Verification items for the finished model (mm, model axes). A direction names the side the tool comes from. Give positions to 0.01 mm unless a question says otherwise; leave off trailing zeros. Loops run counter-clockwise (first coordinate to the right, second up) from the corner with the lowest first, then second, coordinate; pieces in that order, holes last. Notation, with made-up numbers: (23, 3) - (50, 3) arc R21 ccw to (50, 35) - close; hole circle Ø8 at (-2, 53.25). An arc over 180 degrees is marked (long way). Use one line per item in the form item = value.
Autodesk Inventor part; units mm, degrees
ref_plane "YZ Plane" through (0, 0, 0) normal (1, 0, 0) x (0, 1, 0)
ref_plane "XZ Plane" through (0, 0, 0) normal (0, 1, 0) x (-1, 0, 0)
ref_plane "XY Plane" through (0, 0, 0) normal (0, 0, 1) x (1, 0, 0)
sketch "スケッチ1" plane through (0, 0, 0) normal (0, 0, 1) x (1, 0, 0)
  line L0 (-12.5, -43.5) -> (12.5, -43.5)
  line L1 (12.5, -43.5) -> (12.5, 43.5)
  line L2 (12.5, 43.5) -> (-12.5, 43.5)
  line L3 (-12.5, 43.5) -> (-12.5, -43.5)
  line L4 (-12.5, -43.5) -> (12.5, 43.5) construction
  line L5 (12.5, -43.5) -> (-12.5, 43.5) construction
  line L6 (9.6, -40.6) -> (-9.6, -40.6) construction
  line L7 (-9.6, -40.6) -> (-9.6, 40.6) construction
  line L8 (-9.6, 40.6) -> (9.6, 40.6) construction
  line L9 (9.6, 40.6) -> (9.6, -40.6) construction
  line L10 (9.6, -40.6) -> (-9.6, 40.6) construction
  line L11 (-9.6, -40.6) -> (9.6, 40.6) construction
  circle A0 centre (-9.6, -40.6) radius 1.6
  circle A1 centre (-9.6, 40.6) radius 1.6
  circle A2 centre (9.6, 40.6) radius 1.6
  circle A3 centre (9.6, -40.6) radius 1.6
  arc A4 (-7.4091, -42.5) -> (-11.5, -38.4091) centre (-9.6, -40.6) ccw
  line L12 (-7.4091, -42.5) -> (7.4091, -42.5)
  line L13 (0, -43.5) -> (0, 43.5) construction
  line L14 (-12.5, 0) -> (12.5, 0) construction
  arc A5 (11.5, -38.4091) -> (7.4091, -42.5) centre (9.6, -40.6) ccw
  arc A6 (-11.5, 38.4091) -> (-7.4091, 42.5) centre (-9.6, 40.6) ccw
  line L15 (-7.4091, 42.5) -> (7.4091, 42.5)
  arc A7 (7.4091, 42.5) -> (11.5, 38.4091) centre (9.6, 40.6) ccw
  line L16 (-11.5, -38.4091) -> (-11.5, 38.4091)
  line L17 (11.5, -38.4091) -> (11.5, 38.4091)
  point P0 (0, 0)
  dimension "d0" = 25
  dimension "d1" = 87
  dimension "d2" = 19.2
  dimension "d3" = 81.2
  dimension "d4" = 3.2
  dimension "d5" = 1
  dimension "d6" = 1
extrude "押し出し1" add sketch "スケッチ1" along normal blind 1.6 contours L3 L2 L1 L0 | A4 L16 A6 L15 A7 L17 A5 L12
extrude "押し出し2" add sketch "スケッチ1" along normal blind 9.34 contours A4 L16 A6 L15 A7 L17 A5 L12
fillet "フィレット1" radius 2 8 edges at (11.5, -38.4091, 5.47) (7.4091, -42.5, 5.47) (-7.4091, -42.5, 5.47) (-11.5, -38.4091, 5.47) (11.5, 38.4091, 5.47) (7.4091, 42.5, 5.47) (-7.4091, 42.5, 5.47) (-11.5, 38.4091, 5.47)
equation "\"d6\" = d5"
properties part number "IMU-Measurement-and-Transmission-Module"
1. Scan lines: probe 1 along Y at (x, z) = (9.6, 0.8); probe 2 along X at (y, z) = (-1.5, 5); probe 3 along Y at (x, z) = (4, 6). Record each from-to range of solid material in increasing order.
Result set:
probe_1 = -43.5 to -42.2, -39 to 39, 42.2 to 43.5
probe_2 = -11.5 to 11.5
probe_3 = -42.5 to 42.5
2. Tool access check on faces 1 (the cylindrical face through (6.12, 41.91, 5.52)), 2 (the flat face through (0, 42.5, 5)), 3 (the cylindrical face through (-6.12, -41.91, 5.52)). Record the directions out of +Z, -Z, +X, -X, +Y, -Y that give a thin tool (end or side, any length) a straight path to the whole face; none if there is none.
Result set:
face_1 = +Z, +X, +Y
face_2 = +Z, +X, -X, +Y
face_3 = +Z, -X, -Y
3. Draft check along Y on faces 4 (the flat face through (0, 1, 0)), 5 (the flat face through (0, -43.5, 1)), 6 (the cylindrical face through (-9.808, -42.186, 0.789)). Enter one of: released by +Y, released by -Y, zero draft, split by the parting line, or undercut.
Result set:
face_4 = zero draft
face_5 = released by -Y
face_6 = undercut
4. Section check B-B, the plane x = 0.25. Record the cut outline in (y, z).
Result set:
outline = (-43.5, 0) - (43.5, 0) - (43.5, 1.6) - (42.5, 1.6) - (42.5, 9.34) - (-42.5, 9.34) - (-42.5, 1.6) - (-43.5, 1.6) - close
5. Depth check by flat-ended pin: pin 1 Ø4 at (x, y) = (9.6, 40.6) entering from +Z; pin 2 Ø2.5 at (y, z) = (-5, 7) entering from +X; pin 3 Ø2.5 at (x, z) = (-0.5, 5.5) entering from -Y. Enter the tip coordinate at first touch or a pass-through.
Result set:
pin_1 = 1.6
pin_2 = 11.5
pin_3 = -42.5
6. Section check A-A, the plane y = 19.5. Record the cut outline in (x, z).
Result set:
outline = (-12.5, 0) - (12.5, 0) - (12.5, 1.6) - (11.5, 1.6) - (11.5, 9.34) - (-11.5, 9.34) - (-11.5, 1.6) - (-12.5, 1.6) - close
